from build123d import *

# Parameters (mm, degrees)
CROQUIS1_W              = 21.5
CROQUIS1_H              = 26
SALIENTE_EXTRUIR1_DEPTH = 2
CROQUIS2_W              = 46
CROQUIS2_H              = 46
SALIENTE_EXTRUIR2_DEPTH = 2
CROQUIS3_W              = 46
CROQUIS3_H              = 46
CROQUIS3_W_2            = 42
CROQUIS3_H_2            = 42
SALIENTE_EXTRUIR3_DEPTH = 29
CROQUIS4_W              = 42
CROQUIS4_H              = 29
CORTAR_EXTRUIR1_DEPTH   = 29
SALIENTE_EXTRUIR4_DEPTH = 2
CROQUIS6_W              = 2
CROQUIS6_H              = 2
SALIENTE_EXTRUIR5_DEPTH = 30
CROQUIS7_W              = 46
CROQUIS7_H              = 46
SALIENTE_EXTRUIR6_DEPTH = 5
CROQUIS8_R              = 12.5
CORTAR_EXTRUIR2_DEPTH   = 30


with BuildPart() as part:
    # Croquis1 → Saliente-Extruir1 (new body)
    with BuildSketch(Plane(origin=(0, 0, 0), x_dir=(1, 0, 0), z_dir=(0, 1, 0))):
        Rectangle(CROQUIS1_W, CROQUIS1_H)
    extrude(amount=SALIENTE_EXTRUIR1_DEPTH)

    # Croquis2 → Saliente-Extruir2 (add)
    with BuildSketch(Plane.XZ):
        Rectangle(CROQUIS2_W, CROQUIS2_H)
    extrude(amount=SALIENTE_EXTRUIR2_DEPTH)

    # Croquis3 → Saliente-Extruir3 (add)
    with BuildSketch(Plane.XZ.offset(2)):
        Rectangle(CROQUIS3_W, CROQUIS3_H)
        Rectangle(CROQUIS3_W_2, CROQUIS3_H_2, mode=Mode.SUBTRACT)
    extrude(amount=SALIENTE_EXTRUIR3_DEPTH)

    # Croquis4 → Cortar-Extruir1 (cut)
    with BuildSketch(Plane(origin=(23, 0, 0), x_dir=(0, 0, -1), z_dir=(1, 0, 0))):
        with Locations((0, -16.5)):
            Rectangle(CROQUIS4_W, CROQUIS4_H)
    extrude(amount=-CORTAR_EXTRUIR1_DEPTH, mode=Mode.SUBTRACT)

    # Croquis5 → Saliente-Extruir4 (add)
    with BuildSketch(Plane.XZ.offset(31)):
        Polygon((23, 17), (-17, 17), (-17, -17), (23, -17), (23, -23), (-23, -23), (-23, 23), (23, 23), align=None)
    extrude(amount=-SALIENTE_EXTRUIR4_DEPTH)

    # Croquis6 → Saliente-Extruir5 (add)
    with BuildSketch(Plane.XZ.offset(31)):
        with Locations((-22, 22)):
            Rectangle(CROQUIS6_W, CROQUIS6_H)
        with Locations((22, 22)):
            Rectangle(CROQUIS6_W, CROQUIS6_H)
        with Locations((-22, -22)):
            Rectangle(CROQUIS6_W, CROQUIS6_H)
        with Locations((22, -22)):
            Rectangle(CROQUIS6_W, CROQUIS6_H)
    extrude(amount=SALIENTE_EXTRUIR5_DEPTH)

    # Croquis7 → Saliente-Extruir6 (add)
    with BuildSketch(Plane.XZ.offset(61)):
        Rectangle(CROQUIS7_W, CROQUIS7_H)
    extrude(amount=-SALIENTE_EXTRUIR6_DEPTH)

    # Croquis8 → Cortar-Extruir2 (cut)
    with BuildSketch(Plane.XZ.offset(61)):
        with Locations(Location((0, 0, 0), (0, 0, 270))):
            Circle(CROQUIS8_R)
    extrude(amount=-CORTAR_EXTRUIR2_DEPTH, mode=Mode.SUBTRACT)


solid = part.part
Work out the finished part from the listing and answer in its coordinate system (mm). A direction names the side the tool comes from. Give positions to 0.01 mm unless a question says otherwise; leave off trailing zeros. Order: outer loops, then holes, each group sorted by start corner. A loop starts at its lowest first (then second) coordinate and runs counter-clockwise, first axis right, second up. Notation, with made-up numbers: (18.25, 45.25) -> (22.25, 45.25) arc R18 ccw to (22.25, 76.25) -> close; hole circle Ø10 at (-29, 64). An arc over 180 degrees is marked (long way). One line per item, written item: value.
Item 1: Find section C-C, the plane z = -18.5. Give the vertices of the cut face in (x, y).
Answer sheet:
outline: (-23, -61) -> (23, -61) -> (23, -56) -> (-23, -56) -> close; (-23, -31) -> (23, -31) -> (23, -29) -> (-21, -29) -> (-21, -2) -> (23, -2) -> (23, 0) -> (-23, 0) -> close
Item 2: Flat-ended cylindrical pins translate along their axes: P1, Ø5, axis at x = 11, z = 4, coming from the +Y side; P2, Ø4, axis at x = -18, z = -10, coming from the +Y side; P3, Ø6, axis at y = -21.5, z = 8, coming from the +X side. Find the tip coordinate at first contact, or state that the pin passes through.
Answer sheet:
P1: y = 2
P2: y = 0
P3: x = -21
Item 3: Find section A-A, the plane x = -18. Give the vertices of the cut face in (y, z), plus the area to 3 significant figures.
Answer sheet:
outline: (-61, -23) -> (-56, -23) -> (-56, 23) -> (-61, 23) -> close; (-31, -23) -> (0, -23) -> (0, 23) -> (-31, 23) -> close; hole (-29, -21) -> (-2, -21) -> (-2, 21) -> (-29, 21) -> close
area: 522 mm²
Item 4: Find section B-B, the plane z = 0. Give the vertices of the cut face in (x, y), plus the area to 3 significant figures.
Answer sheet:
outline: (-23, -61) -> (-12.5, -61) -> (-12.5, -56) -> (-23, -56) -> close; (-23, -31) -> (-17, -31) -> (-17, -29) -> (-21, -29) -> (-21, -2) -> (23, -2) -> (23, 0) -> (10.75, 0) -> (10.75, 2) -> (-10.75, 2) -> (-10.75, 0) -> (-23, 0) -> close; (12.5, -61) -> (23, -61) -> (23, -56) -> (12.5, -56) -> close
area: 306 mm²
Item 5: Straight lines are drawn through the part: probe 1 along Y at (x, z) = (-14, 6.5); probe 2 along Z at (x, y) = (14.5, -19); probe 3 along X at (y, z) = (-57.3, 0). For each, find the intervals that lie inside material, in ascending order.
Answer sheet:
probe 1: -61 to -56, -2 to 0
probe 2: -23 to -21, 21 to 23
probe 3: -23 to -12.5, 12.5 to 23
Item 6: Determine the mould class of faces 1 (the cylindrical face through (3.755, -58.535, -11.923)), 2 (the flat face through (-11, -61, -10)), 3 (the flat face through (22, -43, 21)) for opening direction Y: released by +Y, released by -Y, zero draft, split by the parting line, or undercut.
Answer sheet:
face 1: zero draft
face 2: released by -Y
face 3: undercut
Item 7: Find section D-D, the plane x = 0. Give the vertices of the cut face in (y, z).
Answer sheet:
outline: (-61, -23) -> (-56, -23) -> (-56, -12.5) -> (-61, -12.5) -> close; (-61, 12.5) -> (-56, 12.5) -> (-56, 23) -> (-61, 23) -> close; (-31, -23) -> (0, -23) -> (0, -13) -> (2, -13) -> (2, 13) -> (0, 13) -> (0, 23) -> (-31, 23) -> (-31, 17) -> (-29, 17) -> (-29, 21) -> (-2, 21) -> (-2, -21) -> (-29, -21) -> (-29, -17) -> (-31, -17) -> close
Item 8: A tool of negligible diameter and unlimited length cuts with its end or side. For faces 4 (the flat face through (-10.75, 1, 0)), 5 (the flat face through (1, -16, 21)), 6 (the flat face through (10.75, 1, 0)), 7 (the flat face through (0, 1, 13)), from which of +Z, -Z, +X, -X, +Y, -Y can it reach the whole face along a straight path? Write none if from no direction.
Answer sheet:
face 4: +Z, -Z, -X, +Y
face 5: +X
face 6: +Z, -Z, +X, +Y
face 7: +Z, +X, -X, +Y
